Work out the finished part from the listing and answer in its coordinate system (mm). A direction names the side the tool comes from. Coordinates: 2 decimals unless noted, no trailing zeros. Loops run counter-clockwise (first coordinate to the right, second up) from the corner with the lowest first, then second, coordinate; pieces in that order, holes last.
```python
from build123d import *

# Parameters (mm, degrees)
CROQUIS1_W                           = 1.5
CROQUIS1_H                           = 1.5
SALIENTE_EXTRUIR1_DEPTH              = 0.5
CROQUIS2_R                           = 1.125
SALIENTE_EXTRUIR2_DEPTH              = 1.25
CROQUIS5_R                           = 2.5
SALIENTE_EXTRUIR5_DEPTH              = 1.5
CROQUIS6_R                           = 1.25
SALIENTE_EXTRUIR6_DEPTH              = 0.25
CROQUIS7_R                           = 0.5
SALIENTE_EXTRUIR7_DEPTH              = 0.5
CORTAR_EXTRUIR1_DEPTH                = 10
TALADRO_ROSCADO_M1X0_251_D           = 0.75
TALADRO_ROSCADO_M1X0_251_DEPTH       = 2.25
TALADRO_ROSCADO_M1X0_251_CBORE_D     = 1
TALADRO_ROSCADO_M1X0_251_CBORE_DEPTH = 2
TALADRO_ROSCADO_M1X0_251_TIP         = 0.225322732


with BuildPart() as part:
    # Croquis1 → Saliente-Extruir1 (new body)
    with BuildSketch(Plane.XY):
        Rectangle(CROQUIS1_W, CROQUIS1_H)
    extrude(amount=SALIENTE_EXTRUIR1_DEPTH)

    # Croquis2 → Saliente-Extruir2 (add)
    with BuildSketch(Plane(origin=(0, 0, 0), x_dir=(-1, 0, 0), z_dir=(0, 0, -1))):
        Circle(CROQUIS2_R)
    extrude(amount=SALIENTE_EXTRUIR2_DEPTH)

    # Croquis5 → Saliente-Extruir5 (add)
    with BuildSketch(Plane(origin=(0, 0, -1.25), x_dir=(-1, 0, 0), z_dir=(0, 0, -1))):
        Circle(CROQUIS5_R)
    extrude(amount=SALIENTE_EXTRUIR5_DEPTH)

    # Croquis6 → Saliente-Extruir6 (add)
    with BuildSketch(Plane(origin=(0, 0, -2.75), x_dir=(-1, 0, 0), z_dir=(0, 0, -1))):
        Circle(CROQUIS6_R)
    extrude(amount=SALIENTE_EXTRUIR6_DEPTH)

    # Croquis7 → Saliente-Extruir7 (add)
    with BuildSketch(Plane(origin=(0, 0, -3), x_dir=(-1, 0, 0), z_dir=(0, 0, -1))):
        Circle(CROQUIS7_R)
    extrude(amount=SALIENTE_EXTRUIR7_DEPTH)

    # Croquis11 → Cortar-Extruir1 (cut)
    with BuildSketch(Plane(origin=(0, 2.25, 0), x_dir=(-1, 0, 0), z_dir=(0, 1, 0))):
        Polygon((-1.5, -1.25), (1.5, -1.25), (1.5, -1.75), (0, -1.75), (0, -2.25), (1.5, -2.25), (1.5, -2.75), (-1.5, -2.75), align=None)
    extrude(amount=CORTAR_EXTRUIR1_DEPTH, mode=Mode.SUBTRACT)

    # Taladro roscado M1x0.251
    with Locations(Plane.XY.offset(0.5)):
        with Locations((0, 0)):
            CounterBoreHole(TALADRO_ROSCADO_M1X0_251_D / 2, TALADRO_ROSCADO_M1X0_251_CBORE_D / 2, TALADRO_ROSCADO_M1X0_251_CBORE_DEPTH, depth=TALADRO_ROSCADO_M1X0_251_DEPTH)
            with Locations((0, 0, -(TALADRO_ROSCADO_M1X0_251_DEPTH + TALADRO_ROSCADO_M1X0_251_TIP / 2))):  # 118° drill point
                Cone(0, TALADRO_ROSCADO_M1X0_251_D / 2, TALADRO_ROSCADO_M1X0_251_TIP, mode=Mode.SUBTRACT)


solid = part.part
```
1. A cutting plane is placed at C-C, the plane x = 2. Give the vertices of the cut face in (y, z).
2. For faces 4 (the flat face through (0, 0, -3.5)), 5 (the flat face through (-1, -1, -1.25)), 6 (the flat face through (-1, -1, -2.75)), determine the directions among +Z, -Z, +X, -X, +Y, -Y from which every point of the face is accessible in a straight line to the end or side of a thin tool.
3. Straight lines are drawn through the part: probe 1 along X at (y, z) = (0, -1.6) (3 decimals); probe 2 along Y at (x, z) = (0, -0.1) (3 decimals); probe 3 along Y at (x, z) = (0, -1.55) (3 decimals). For each, find the intervals that lie inside material, in ascending order.
4. A cutting plane is placed at A-A, the plane z = -0.3. Give the vertices of the cut face in (x, y) (3 decimals), then the cut area to 3 significant figures.
5. A cutting plane is placed at B-B, the plane y = 0.6. Give the vertices of the cut face in (x, z), then the cut area to 3 significant figures.
6. A cutting plane is placed at D-D, the plane z = -2.85. Give the vertices of the cut face in (x, y), then the cut area to 3 significant figures.
7. Each of these flat-tipped pins is pushed along its axis until it touches: P1, Ø0.6, axis at x = 0, z = 0, coming from the -Y side (3 decimals); P2, Ø0.6, axis at y = 0, z = 0, coming from the +X side (3 decimals); P3, Ø2.5, axis at x = -1, y = -1, coming from the +Z side; P4, Ø1, axis at y = 1, z = -3, coming from the +X side. Where does it stop, or does it pass through?
8. Determine the mould class of faces 1 (the flat face through (0, -1, -3)), 2 (the cylindrical face through (-0.108, -0.488, -0.486)), 3 (the cylindrical face through (-0.459, -2.457, -1.99)) for opening direction X: released by +X, released by -X, zero draft, split by the parting line, or undercut.
Answers below:
1. outline: (-1.5, -2.75) - (1.5, -2.75) - (1.5, -1.25) - (-1.5, -1.25) - close
2. face 4: -Z, +X, -X, +Y, -Y
2. face 5: +Z
2. face 6: -Z
3. probe 1: x = -2.5 to -0.375, 0.375 to 2.5
3. probe 2: y = -1.125 to -0.5, 0.5 to 1.125
3. probe 3: y = -2.5 to -0.375, 0.375 to 2.25
4. outline: circle Ø2.25 at (0, 0); hole circle Ø1 at (0, 0)
4. area: 3.19 mm2
5. outline: (-2.43, -2.75) - (-1.1, -2.75) - (-1.1, -3) - (1.1, -3) - (1.1, -2.75) - (2.43, -2.75) - (2.43, -1.25) - (0.95, -1.25) - (0.95, 0) - (0.75, 0) - (0.75, 0.5) - (-0.75, 0.5) - (-0.75, 0) - (-0.95, 0) - (-0.95, -1.25) - (-2.43, -1.25) - close
5. area: 11.0 mm2
6. outline: circle Ø2.5 at (0, 0)
6. area: 4.91 mm2
7. P1: stops at y = -1.125
7. P2: stops at x = 1.125
7. P3: stops at z = 0.5
7. P4: stops at x = 2.43
8. face 1: zero draft
8. face 2: undercut
8. face 3: split by the parting line
